Check sheet for the drawn part. Datum: minimum x, y, z corner. Units: mm. Coordinates: 2 decimals unless noted, no trailing zeros. Loops run counter-clockwise (first coordinate to the right, second up) from the corner with the lowest first, then second, coordinate; pieces in that order, holes last.
Q1. Sectioned sample at C-C (x = 20). Enter the section's corners in (y, z).
Q2. Sectioned sample at D-D (z = 4.5). Enter the section's corners in (x, y), then the cut area to 3 significant figures.
Q3. Go/stop test with flat-tipped pins: P1, Ø4, axis at x = 3, z = 5.5, coming from the +Y side; P2, Ø6.5, axis at x = 20, z = 4.5, coming from the -Y side; P3, Ø2, axis at x = 19.5, z = 11.5, coming from the +Y side. Record where each tip stops, or that it passes through.
Q4. Mould release check, pull along Y, two halves, no side actions. Record for the marked faces 1 and 2: +Y half, -Y half, draft (parallel to the pull), parting line (faces both ways), or undercut.
Q5. Material ranges on probe 1 along X at (y, z) = (1.35, 4.5); probe 2 along Y at (x, z) = (3.25, 13.5); probe 3 along X at (y, z) = (1.05, 6), recorded low to high.
Q6. Sectioned sample at B-B (y = 2.5). Enter the section's corners in (x, z).
Q7. Sectioned sample at A-A (z = 13.5). Enter the section's corners in (x, y), then the cut area to 3 significant figures.
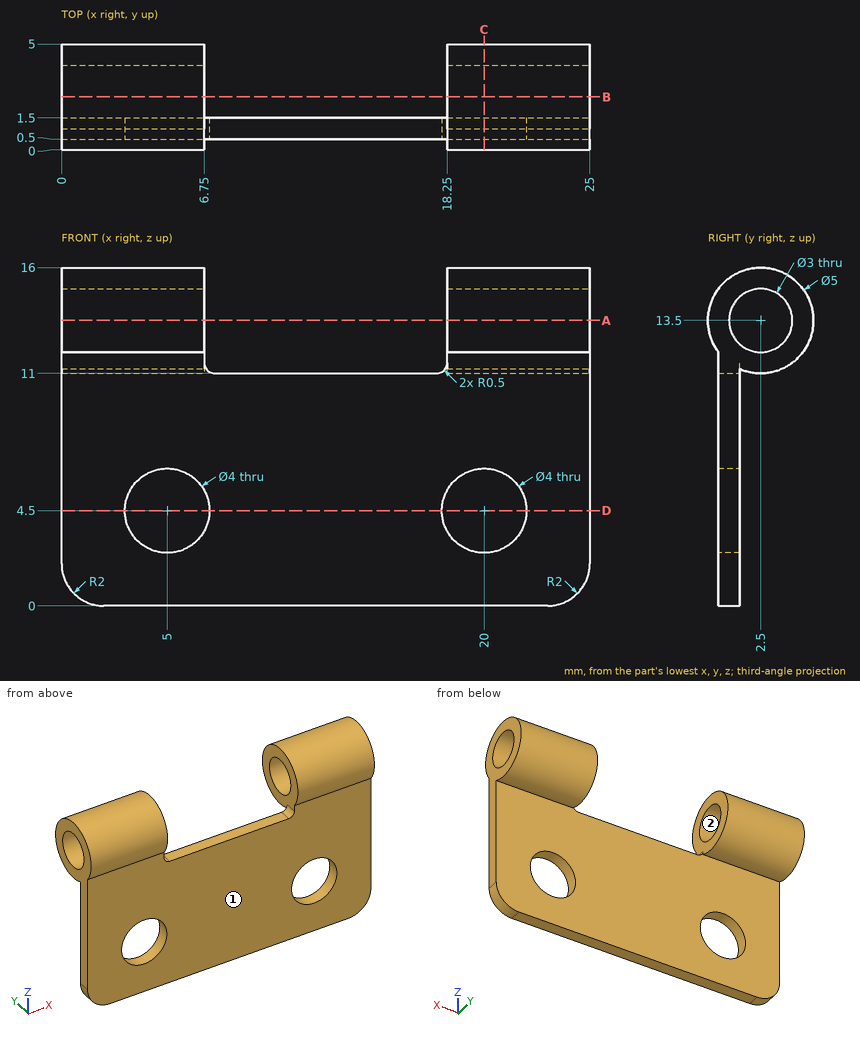
Geometry check:
1. outline: (0.5, 0) - (1.5, 0) - (1.5, 2.5) - (0.5, 2.5) - close; (0.5, 6.5) - (1.5, 6.5) - (1.5, 11.21) arc R2.5 ccw (long way) to (0.5, 12) - close; hole circle Ø3 at (2.5, 13.5)
2. outline: (0, 0.5) - (3, 0.5) - (3, 1.5) - (0, 1.5) - close; (7, 0.5) - (18, 0.5) - (18, 1.5) - (7, 1.5) - close; (22, 0.5) - (25, 0.5) - (25, 1.5) - (22, 1.5) - close
2. area: 17.0 mm2
3. P1: stops at y = 1.5
3. P2: stops at y = 0.5
3. P3: stops at y = 4.79
4. face 1: -Y half
4. face 2: undercut
5. probe 1: x = 0 to 3, 7 to 18, 22 to 25
5. probe 2: y = 0 to 1, 4 to 5
5. probe 3: x = 0 to 3.68, 6.32 to 18.68, 21.32 to 25
6. outline: (0, 11) - (6.75, 11) - (6.75, 12) - (0, 12) - close; (0, 15) - (6.75, 15) - (6.75, 16) - (0, 16) - close; (18.25, 11) - (25, 11) - (25, 12) - (18.25, 12) - close; (18.25, 15) - (25, 15) - (25, 16) - (18.25, 16) - close
7. outline: (0, 0) - (6.75, 0) - (6.75, 1) - (0, 1) - close; (0, 4) - (6.75, 4) - (6.75, 5) - (0, 5) - close; (18.25, 0) - (25, 0) - (25, 1) - (18.25, 1) - close; (18.25, 4) - (25, 4) - (25, 5) - (18.25, 5) - close
7. area: 27.0 mm2
